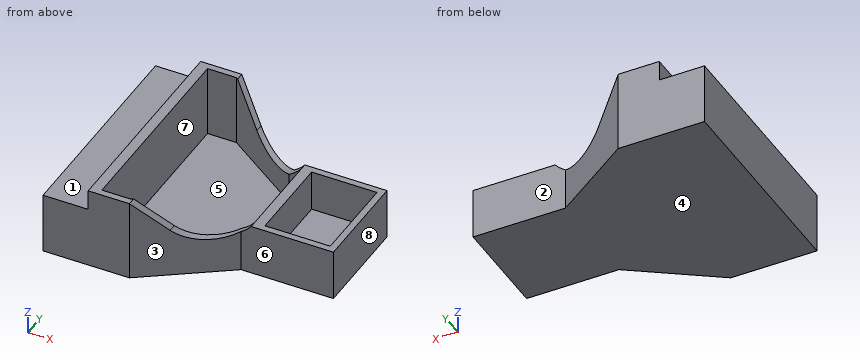
from build123d import *

# Parameters (mm, degrees)
F0_W      = 13.843
F0_H      = 10.0965
F1_DEPTH  = 12.7
F3_DEPTH  = 1.5875
F5_DEPTH  = 33.3385
F6_W      = 33.3375
F6_H      = 9.525
F7_DEPTH  = 6.985
F9_ANGLE  = -90
F11_ANGLE = -90


with BuildPart() as f1:
    # F0 (on Front) → F1 (new body)
    with BuildSketch(Plane.XZ):
        Polygon((7.9375, 33.3375), (-7.9375, 33.3375), (-7.9375, 19.05), (-16.66875, 6.35), (-16.66875, 0), (16.66875, 0), (16.66875, 6.35), (7.9375, 19.05), align=None)
        Polygon((15.65275, 6.0344407596), (15.65275, 1.5875), (-15.65275, 1.5875), (-15.65275, 6.0344407596), (-6.9215, 18.7344407596), (-6.9215, 20.6375), (6.9215, 20.6375), (6.9215, 18.7344407596), align=None, mode=Mode.SUBTRACT)
        with Locations((0, 27.27325)):
            Rectangle(F0_W, F0_H, mode=Mode.SUBTRACT)
    extrude(amount=F1_DEPTH)

    # F2 (on Front) → F3 (join)
    with BuildSketch(Plane.XZ):
        Polygon((7.9375, 33.3375), (-7.9375, 33.3375), (-7.9375, 19.05), (-16.66875, 6.35), (-16.66875, 0), (16.66875, 0), (16.66875, 6.35), (7.9375, 19.05), align=None)
    extrude(amount=F3_DEPTH)

    # F4 (on face) → F5 (cut, through all)
    with BuildSketch(Plane.YZ.offset(16.66875)):
        with BuildLine():
            Line((-12.7, 33.3375), (-12.7, 6.35))
            Line((-12.7, 6.35), (-7.6210542824, 10.9944259619))
            ThreePointArc((-7.6210542824, 10.9944259619), (-5.559666336, 15.8888014069), (-7.9375, 20.6375))
            Line((-7.9375, 20.6375), (-7.9375, 33.3375))
            Line((-7.9375, 33.3375), (-12.7, 33.3375))
        make_face()
    extrude(amount=-F5_DEPTH, mode=Mode.SUBTRACT)

    # F6 (on face) → F7 (join)
    with BuildSketch(Plane(origin=(0, 0, 0), x_dir=(1, 0, 0), z_dir=(0, 0, -1))):
        with Locations((0, 4.7625)):
            Rectangle(F6_W, F6_H)
    extrude(amount=F7_DEPTH)


with BuildPart() as f1_1:
    # F9: moved
    add(f1.part.rotate(Axis((0, 0, -6.985), (1, 0, 0)), F9_ANGLE))


with BuildPart() as f1_2:
    # F11: moved
    add(f1_1.part.rotate(Axis((0, 0, -2.2225), (0, 0, 1)), F11_ANGLE))


with BuildPart() as f1_3:
    # F12: moved
    add(f1_2.part.moved(Location((0, 0, -5.715))))


solid = f1_3.part
Here's how the part is built. I have some questions about the finished solid (model axes, mm). Face numbers are marked on the shaded views. A direction names the side the tool comes from. Round coordinates to 2 decimals unless told otherwise and drop trailing zeros. Loops run counter-clockwise (first coordinate to the right, second up) from the corner with the lowest first, then second, coordinate; pieces in that order, holes last.
1. If I drill on line 1 along X through (y, z) = (2, -9.75); line 2 along Y through (x, z) = (38, -6); line 3 along Z through (x, y) = (3, 15) (3 decimals), over which ranges is the centre line in solid material (lowest first)?
Answer list:
line 1: x = 0 to 8.57, 27.62 to 29.21, 39.31 to 40.32
line 2: y = -7.94 to -6.92, 6.92 to 7.94
line 3: z = -12.7 to -3.175
2. We'd pull the mould along Y, two halves only. Please class the marked faces 6, 7 and 8: +Y half, -Y half, draft (parallel to the pull), parting line (faces both ways), or undercut.
Answer list:
face 6: -Y half
face 7: undercut
face 8: draft
3. Which directions (+Z, -Z, +X, -X, +Y, -Y) give clear straight access to the entire face, cutting with the end or side of a thin tool? Please do the marked faces 1, 2, 3, 4 and 5.
Answer list:
face 1: +Z, -X, +Y, -Y
face 2: +Z, -Z, +X, +Y
face 3: +Z, -Z, +X, -Y
face 4: -Z, +X, -X, +Y, -Y
face 5: +Z
4. If we section it at D-D on z = -0.75: Write out the boundary of the cut face in (x, y) (1 decimal).
Answer list:
outline: (7, -16.7) - (13.3, -16.7) - (14, -16.2) - (14, -15) - (13, -15.7) - (8.6, -15.7) - (8.6, 15.7) - (13, 15.7) - (14, 15) - (14, 16.2) - (13.3, 16.7) - (7, 16.7) - close
5. If we section it at A-A on z = -10.25: Write out the boundary of the cut face in (x, y) (1 decimal), plus the area to 3 significant figures.
Answer list:
outline: (0, -16.7) - (13.3, -16.7) - (26, -7.9) - (40.3, -7.9) - (40.3, 7.9) - (26, 7.9) - (13.3, 16.7) - (0, 16.7) - close; hole (8.6, -15.7) - (13, -15.7) - (25.7, -6.9) - (27.6, -6.9) - (27.6, 6.9) - (25.7, 6.9) - (13, 15.7) - (8.6, 15.7) - close; hole (29.2, -6.9) - (39.3, -6.9) - (39.3, 6.9) - (29.2, 6.9) - close
area: 392 mm2
6. For P1, Ø1.9, axis at x = 32, z = -6.5, coming from the +Y side; P2, Ø3.5, axis at x = 3, y = 7, coming from the +Z side (3 decimals); P3, Ø7, axis at x = 34.5, z = -8, coming from the -Y side; P4, Ø2, axis at x = 29, y = -9, coming from the +Z side, each with a flat end and sliding along its axis, tell me the tip position at first contact or that it passes through.
Answer list:
P1: stops at y = 7.94
P2: stops at z = -3.175
P3: stops at y = -7.94
P4: passes through
7. If we section it at B-B on x = 36.5: Write out the boundary of the cut face in (y, z).
Answer list:
outline: (-7.94, -12.7) - (7.94, -12.7) - (7.94, -4.76) - (6.92, -4.76) - (6.92, -11.11) - (-6.92, -11.11) - (-6.92, -4.76) - (-7.94, -4.76) - close
